Check sheet for the modelled part. Datum: model origin and axes. Units: mm. Face numbers are marked on the shaded views. A direction names the side the tool comes from. Give positions to 0.01 mm unless a question says otherwise; leave off trailing zeros. Order: outer loops, then holes, each group sorted by start corner. A loop starts at its lowest first (then second) coordinate and runs counter-clockwise, first axis right, second up.
Autodesk Inventor part; units mm, degrees
ref_plane "YZ Plane" through (0, 0, 0) normal (1, 0, 0) x (0, 1, 0)
ref_plane "XZ Plane" through (0, 0, 0) normal (0, 1, 0) x (-1, 0, 0)
ref_plane "XY Plane" through (0, 0, 0) normal (0, 0, 1) x (1, 0, 0)
sketch "Sketch1" plane through (0, 0, 0) normal (0, 1, 0) x (-1, 0, 0)
  line L0 (0, 0) -> (50.8, 0)
  line L1 (50.8, 0) -> (50.8, -203.2)
  line L2 (50.8, -203.2) -> (0, -203.2)
  line L3 (0, -203.2) -> (0, 0)
  dimension "d0" = 50.8
  dimension "d1" = 203.2
extrude "Extrusion1" add sketch "Sketch1" along normal blind 25.4
sketch "Sketch2" plane through (0, 25.4, 0) normal (0, 1, 0) x (1, 0, 0)
  line L0 (-50.8, 0) -> (0, 0)
  line L1 (0, 0) -> (0, 203.2)
  line L2 (-50.8, 0) -> (0, 0)
  line L3 (0, 0) -> (0, 25.4)
  line L4 (0, 25.4) -> (-50.8, 25.4)
  line L5 (-50.8, 25.4) -> (-50.8, 0)
  dimension "d4" = 25.4
extrude "Extrusion2" add sketch "Sketch2" along normal blind 330.2
sketch "Sketch3" plane through (0, 355.6, 0) normal (0, 1, 0) x (1, 0, 0)
  line L0 (0, 203.2) -> (-50.8, 203.2)
  line L1 (0, 0) -> (-50.8, 0)
  line L2 (-50.8, 0) -> (-50.8, 203.2)
  line L3 (-50.8, 203.2) -> (0, 203.2)
  line L4 (0, 203.2) -> (0, 0)
extrude "Extrusion3" add sketch "Sketch3" along normal blind 25.4
sketch "Sketch4" plane through (-50.8, 0, 0) normal (0, 0, 1) x (1, 0, 0)
  line L0 (50.8, 292.1) -> (25.4, 292.1)
  line L1 (25.4, 292.1) -> (25.4, 266.7)
  line L2 (25.4, 266.7) -> (50.8, 266.7)
  line L3 (50.8, 266.7) -> (50.8, 292.1)
  line L4 (50.8, 88.9) -> (25.4, 88.9)
  line L5 (25.4, 88.9) -> (25.4, 114.3)
  line L6 (25.4, 114.3) -> (50.8, 114.3)
  line L7 (50.8, 114.3) -> (50.8, 88.9)
  line L8 (50.8, 0) -> (0, 0)
  dimension "d19" = 152.4
  dimension "d20" = 25.4
  dimension "d21" = 25.4
  dimension "d22" = 88.9
extrude "Extrusion4" add sketch "Sketch4" along normal blind 38.1
sketch "Sketch6" plane through (-25.4, 114.3, 0) normal (0, 1, 0) x (1, 0, 0)
  circle A0 centre (12.7, -25.4) radius 12.7
  line L0 (25.4, 0) -> (25.4, -38.1)
  line L1 (25.4, -38.1) -> (0, -38.1)
  dimension "d23" = 25.4
  dimension "d24" = 12.7
  dimension "d25" = 12.7
extrude "Extrusion5" add sketch "Sketch6" along normal blind 158.75 contours A0
properties part number "hand"
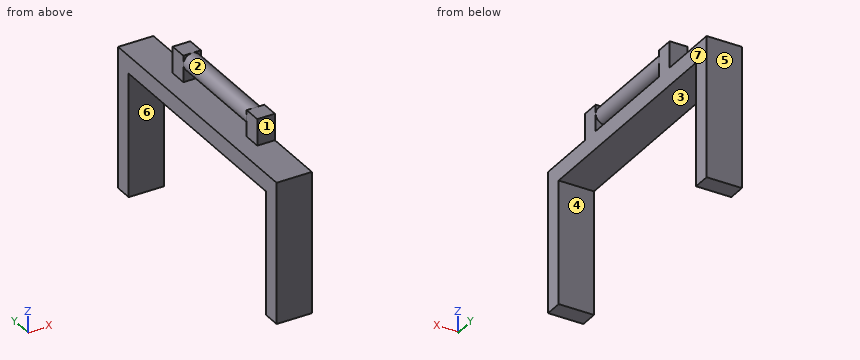
(1) Cross-section at C-C on x = -31. Enter the section's corners in (y, z), then the cut area to 3 significant figures.
Response values:
outline: (0, -203.2) - (25.4, -203.2) - (25.4, -25.4) - (355.6, -25.4) - (355.6, -203.2) - (381, -203.2) - (381, 0) - (0, 0) - close
area: 18,700 mm2
(2) Cross-section at D-D on z = -38.5. Enter the section's corners in (x, y).
Response values:
outline: (-50.8, 0) - (0, 0) - (0, 25.4) - (-50.8, 25.4) - close; (-50.8, 355.6) - (0, 355.6) - (0, 381) - (-50.8, 381) - close
(3) Cross-section at A-A on z = 9. Enter the section's corners in (x, y).
Response values:
outline: (-25.4, 88.9) - (0, 88.9) - (0, 114.3) - (-25.4, 114.3) - close; (-25.4, 266.7) - (0, 266.7) - (0, 292.1) - (-25.4, 292.1) - close
(4) Cross-section at B-B on y = 203.5. Enter the section's corners in (x, z), then the cut area to 3 significant figures.
Response values:
outline: (-50.8, -25.4) - (0, -25.4) - (0, 0) - (-50.8, 0) - close; circle Ø25.4 at (-12.7, 25.4)
area: 1,800 mm2
(5) Material ranges on L1, parallel to Y at x = -7, z = -101.5; L2, parallel to Z at x = -20.5, y = 337; L3, parallel to Z at x = -17, y = 94, recorded low to high.
Response values:
L1: y = 0 to 25.4, 355.6 to 381
L2: z = -25.4 to 0
L3: z = -25.4 to 38.1
(6) Set-up check for the marked faces 1, 2 and 3: record each of +Z, -Z, +X, -X, +Y, -Y from which the full face is reachable in a straight line by a thin tool's end or side.
Response values:
face 1: +Z, +X, -X, -Y
face 2: none
face 3: -Z, +X, -X
(7) Gauge pin test, flat ends, axial feed: pin 1 Ø14 at (x, z) = (-17.5, 31.5) entering from -Y; pin 2 Ø10 at (x, z) = (-16.5, 32.5) entering from +Y; pin 3 Ø3 at (x, y) = (-18, 128.5) entering from -Z. Record the tip position at first contact, or that the pin passes through.
Response values:
pin 1: stops at y = 88.9
pin 2: stops at y = 292.1
pin 3: stops at z = -25.4
(8) Release check for a two-part mould opening along Y. For the marked faces 4, 5, 6 and 7 record: released by +Y, released by -Y, zero draft, split by the parting line, or undercut.
Response values:
face 4: undercut
face 5: released by +Y
face 6: undercut
face 7: zero draft
